Could you check a few things on this model? Use its own coordinates, in mm. Face numbers are marked on the shaded views. A direction names the side the tool comes from. Round coordinates to 2 decimals unless told otherwise and drop trailing zeros. Write each loop counter-clockwise with the first axis right and the second up, starting at its lowest first coordinate (ties: lowest second). Pieces come first, ordered by that corner, then holes. Notation, with made-up numbers: (-12.75, 51.25) -> (38.25, 51.25) arc R24 cw to (38.25, 75.25) -> close; hole circle Ø7 at (13.5, 30). An arc over 180 degrees is marked (long way). Return JSON: item names as keys, results as strings.
from build123d import *

# Parameters (mm, degrees)
SKETCH_1_R                      = 17.5
SKETCH_1_R_2                    = 12.5
CUT_EXTRUDE_3_REACH             = 483.521
SKETCH_3_R                      = 17.5
SKETCH_3_R_2                    = 12.5
CUT_EXTRUDE_3_DIRECTION_2_DEPTH = 150


with BuildPart() as part:
    # Sweep 1: sweep along a path in Sketch 2
    with BuildLine(Plane(origin=(0, 0, 0), x_dir=(1, 0, 0), z_dir=(0, 1, 0))) as sweep_1_path:
        Line((0, 0), (-450, 0))
        ThreePointArc((-450, 0), (-485.355339059, 14.644660941), (-500, 50))
        Line((-500, 50), (-500, 400))
    # Sketch 1 → Sweep 1 (sweep)
    with BuildSketch(Plane(origin=(0, 0, 0), x_dir=(0, 0, -1), z_dir=(1, 0, 0))):
        Circle(SKETCH_1_R)
        Circle(SKETCH_1_R_2, mode=Mode.SUBTRACT)
    sweep(path=sweep_1_path.line)

    # Sketch 3 → Cut-Extrude 3 (cut, up to next)
    with BuildSketch(Plane(origin=(-250, 0, 0), x_dir=(0, 0, -1), z_dir=(1, 0, 0)), mode=Mode.PRIVATE) as cut_extrude_3_sk1:
        with Locations(Location((0, 0, 0), (0, 0, 180))):
            Circle(SKETCH_3_R)
        with Locations(Location((0, 0, 0), (0, 0, 180))):
            Circle(SKETCH_3_R_2, mode=Mode.SUBTRACT)
    cut_extrude_3_tool1 = extrude(cut_extrude_3_sk1.sketch, amount=CUT_EXTRUDE_3_REACH, mode=Mode.PRIVATE) & part.part
    add(cut_extrude_3_tool1.solids().sort_by_distance((-250, 0, -17.005025))[0], mode=Mode.SUBTRACT)

    # Sketch 3 → Cut-Extrude 3 direction 2 (cut)
    with BuildSketch(Plane(origin=(-250, 0, 0), x_dir=(0, 0, -1), z_dir=(1, 0, 0))):
        with Locations(Location((0, 0, 0), (0, 0, 180))):
            Circle(SKETCH_3_R)
        with Locations(Location((0, 0, 0), (0, 0, 180))):
            Circle(SKETCH_3_R_2, mode=Mode.SUBTRACT)
    extrude(amount=-CUT_EXTRUDE_3_DIRECTION_2_DEPTH, mode=Mode.SUBTRACT)


solid = part.part
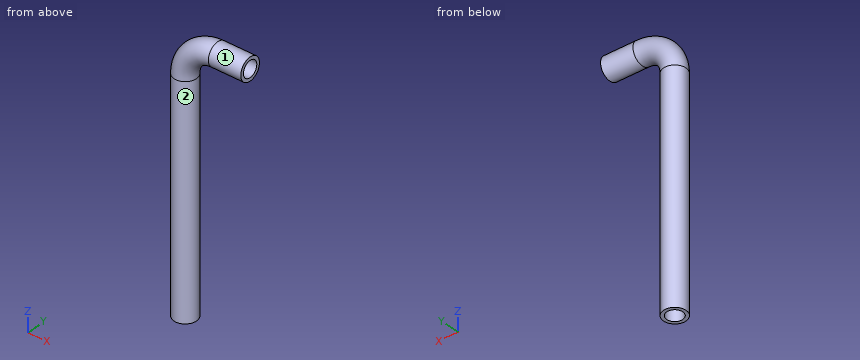
1) I want a section at A-A, the plane y = 0. Please give me the cut outline in (x, z), and give its area (3 significant figures).
Return value:
{"outline": "(-517.5, -400) -> (-512.5, -400) -> (-512.5, -50) arc R62.5 cw to (-450, 12.5) -> (-400, 12.5) -> (-400, 17.5) -> (-450, 17.5) arc R67.5 ccw to (-517.5, -50) -> close; (-487.5, -400) -> (-482.5, -400) -> (-482.5, -50) arc R32.5 cw to (-450, -17.5) -> (-400, -17.5) -> (-400, -12.5) -> (-450, -12.5) arc R37.5 ccw to (-487.5, -50) -> close", "area": "4,790 mm²"}
2) Will these pins go through, and if not, where does the flat tip stop? pin 1 Ø6 at (y, z) = (11, -93) entering from -X; pin 2 Ø8 at (x, y) = (-431.5, 10) entering from +Z; pin 3 Ø6 at (y, z) = (-11.5, -58) entering from +X.
Return value:
{"pin 1": "x = -515.56", "pin 2": "z = 16.44", "pin 3": "x = -484.7"}
3) I want a section at C-C, the plane x = -424. Please give me the cut outline in (y, z).
Return value:
{"outline": "circle Ø35 at (0, 0); hole circle Ø25 at (0, 0)"}
4) For the marked faces 1 and 2, which set-ups out of +Z, -Z, +X, -X, +Y, -Y let a thin tool reach every point of the face, with its end or its side?
Return value:
{"face 1": "+X", "face 2": "-Z"}
5) If I drill on probe 1 along Z at (x, y) = (-417, 0); probe 2 along X at (y, z) = (-0.5, -61.5), over which ranges is the centre line in solid material (lowest first)? Write a range as [from, to].
Return value:
{"probe 1": "[-17.5, -12.5], [12.5, 17.5]", "probe 2": "[-517.49, -512.49], [-487.51, -482.51]"}
6) I want a section at B-B, the plane z = -310. Please give me the cut outline in (x, y).
Return value:
{"outline": "circle Ø35 at (-500, 0); hole circle Ø25 at (-500, 0)"}
